```python
from build123d import *

# Parameters (mm, degrees)
SKETCH_W     = 19.8
SKETCH_H     = 11.5
PAD_DEPTH    = 6.4
SKETCH001_R  = 1.2
POCKET_DEPTH = 6.401
SKETCH002_W  = 1
SKETCH002_H  = 3.2
PAD001_DEPTH = 3.5


with BuildPart() as part:
    # Sketch → Pad (new body)
    with BuildSketch(Plane.XY):
        with Locations((9.9, 5.75)):
            Rectangle(SKETCH_W, SKETCH_H)
    extrude(amount=PAD_DEPTH)

    # Sketch001 → Pocket (cut, through all)
    with BuildSketch(Plane.XY.offset(6.4)):
        with Locations((4.8, 2.9)):
            Circle(SKETCH001_R)
        with Locations((15, 2.9)):
            Circle(SKETCH001_R)
    extrude(amount=-POCKET_DEPTH, mode=Mode.SUBTRACT)

    # Sketch002 → Pad001 (new body)
    with BuildSketch(Plane.XZ):
        with Locations((1.85, 3.1)):
            Rectangle(SKETCH002_W, SKETCH002_H)
        with Locations((10.65, 3.1)):
            Rectangle(SKETCH002_W, SKETCH002_H)
        with Locations((17.95, 3.1)):
            Rectangle(SKETCH002_W, SKETCH002_H)
    extrude(amount=PAD001_DEPTH)


solid = part.part
```
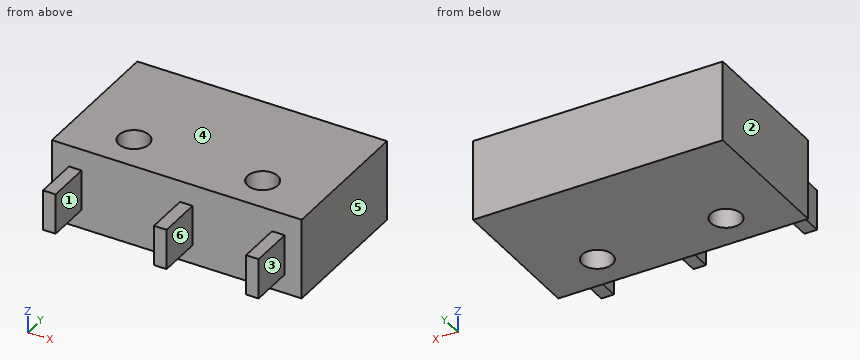
Can you work these out from the model? Positions are in its coordinate system, mm. Face numbers are marked on the shaded views. A direction names the side the tool comes from. Give positions to 0.01 mm unless a question says otherwise; leave off trailing zeros. Order: outer loops, then holes, each group sorted by start corner. A loop starts at its lowest first (then second) coordinate and runs counter-clockwise, first axis right, second up. Notation, with made-up numbers: M 76,23.5 L 87,23.5 A30 cw 87,46.5 Z; hole C 73.25,-34.75 d4. An arc over 180 degrees is marked long. One line per item, written item: value.
1) I want a section at D-D, the plane x = 4. List the corners of the cut face in (y, z) for me, plus the area to 3 significant figures.
Answer sheet:
outline: M 0,0 L 2.01,0 L 2.01,6.4 L 0,6.4 Z; M 3.79,0 L 11.5,0 L 11.5,6.4 L 3.79,6.4 Z
area: 62.2 mm^2
2) Please list where these lines run through material, in increasing order: line 1 along X through (y, z) = (2.75, 5.25); line 2 along Y through (x, z) = (4.8, 4.5); line 3 along Y through (x, z) = (9.5, 4.5).
Answer sheet:
line 1: x = 0 to 3.61, 5.99 to 13.81, 16.19 to 19.8
line 2: y = 0 to 1.7, 4.1 to 11.5
line 3: y = 0 to 11.5
3) For P1, Ø3.5, axis at y = -2, z = 3.5, coming from the +X side; P2, Ø3.5, axis at y = -2, z = 3, coming from the -X side; P3, Ø1.5, axis at x = 2.5, y = -1, coming from the -Z side, each with a flat end and sliding along its axis, tell me the tip position at first contact or that it passes through.
Answer sheet:
P1: stops at x = 18.45
P2: stops at x = 1.35
P3: stops at z = 1.5
4) I want a section at B-B, the plane x = 15. List the corners of the cut face in (y, z) for me.
Answer sheet:
outline: M 0,0 L 1.7,0 L 1.7,6.4 L 0,6.4 Z; M 4.1,0 L 11.5,0 L 11.5,6.4 L 4.1,6.4 Z
5) I want a section at C-C, the plane z = 3. List the corners of the cut face in (x, y) for me, plus the area to 3 significant figures.
Answer sheet:
outline: M 0,0 L 1.35,0 L 1.35,-3.5 L 2.35,-3.5 L 2.35,0 L 10.15,0 L 10.15,-3.5 L 11.15,-3.5 L 11.15,0 L 17.45,0 L 17.45,-3.5 L 18.45,-3.5 L 18.45,0 L 19.8,0 L 19.8,11.5 L 0,11.5 Z; hole C 4.8,2.9 d2.4; hole C 15,2.9 d2.4
area: 229 mm^2
6) I want a section at A-A, the plane y = -0.25. List the corners of the cut face in (x, z) for me.
Answer sheet:
outline: M 1.35,1.5 L 2.35,1.5 L 2.35,4.7 L 1.35,4.7 Z; M 10.15,1.5 L 11.15,1.5 L 11.15,4.7 L 10.15,4.7 Z; M 17.45,1.5 L 18.45,1.5 L 18.45,4.7 L 17.45,4.7 Z
7) We'd pull the mould along X, two halves only. Please class the marked faces 4, 5 and 6: released by +X, released by -X, zero draft, split by the parting line, or undercut.
Answer sheet:
face 4: zero draft
face 5: released by +X
face 6: undercut
8) On a 3-axis mill with a long thin cutter (end or side, diameter ignored), from which of +Z, -Z, +X, -X, +Y, -Y can I reach the whole of each face in a straight line? I mean the marked faces 1, 2 and 3. Say none if no direction works.
Answer sheet:
face 1: +Z, -Z, -Y
face 2: +Z, -Z, -X, +Y, -Y
face 3: +Z, -Z, +X, -Y
